For this review, take the finished solid that the model builds, in its own axes (mm). A direction names the side the tool comes from. Coordinates: 2 decimals unless noted, no trailing zeros. Loops run counter-clockwise (first coordinate to the right, second up) from the corner with the lowest first, then second, coordinate; pieces in that order, holes last. Notation, with made-up numbers: (-11, 2.25) -> (4, 2.25) arc R34 cw to (4, 41.25) -> close; hole circle Ø10 at (-21.75, 6). An arc over 180 degrees is marked (long way). Use a Markdown table: item, result.
from build123d import *

# Parameters (mm, degrees)
SKETCH1_R           = 4
BOSS_EXTRUDE1_DEPTH = 5
BOSS_EXTRUDE2_DEPTH = 35
SKETCH1_4_W         = 5
SKETCH1_4_H         = 35
BOSS_EXTRUDE3_DEPTH = 20
CHAMFER1_SIZE       = 8
CHAMFER1_SIZE2      = 21
FILLET1_R           = 25


with BuildPart() as part:
    # Sketch1 → Boss-Extrude1 (new body)
    with BuildSketch(Plane(origin=(0, 0, 0), x_dir=(1, 0, 0), z_dir=(0, 1, 0))):
        Polygon((5, -5), (5, -40), (60, -40), (75, -25), (75, -5), align=None)
        with Locations(Location((20, -25, 0), (0, 0, 270))):
            Circle(SKETCH1_R, mode=Mode.SUBTRACT)
        with Locations(Location((55, -25, 0), (0, 0, 270))):
            Circle(SKETCH1_R, mode=Mode.SUBTRACT)
    extrude(amount=BOSS_EXTRUDE1_DEPTH)

    # Sketch1_3 → Boss-Extrude2 (add)
    with BuildSketch(Plane(origin=(0, 0, 0), x_dir=(1, 0, 0), z_dir=(0, 1, 0))):
        Polygon((0, -5), (5, -5), (75, -5), (75, 0), (0, 0), align=None)
    extrude(amount=BOSS_EXTRUDE2_DEPTH)

    # Sketch1_4 → Boss-Extrude3 (add)
    with BuildSketch(Plane(origin=(0, 0, 0), x_dir=(1, 0, 0), z_dir=(0, 1, 0))):
        with Locations((2.5, -22.5)):
            Rectangle(SKETCH1_4_W, SKETCH1_4_H)
    extrude(amount=BOSS_EXTRUDE3_DEPTH)

    # Chamfer1
    chamfer1_edges = [part.edges().sort_by_distance(p)[0] for p in [
        (2.5, 20, 40),
    ]]
    chamfer1_side = [part.faces().sort_by_distance(p)[0] for p in [
        (24.5, 4.5, 40),
    ]]
    chamfer(chamfer1_edges, length=CHAMFER1_SIZE, length2=CHAMFER1_SIZE2, reference=chamfer1_side[0])

    # Fillet1
    fillet1_edges = [part.edges().sort_by_distance(p)[0] for p in [
        (75, 35, 2.5),
    ]]
    fillet(fillet1_edges, radius=FILLET1_R)


solid = part.part
(1) Mouldability with a two-part tool opening along X and no side actions: class faces 4 (the face through (40, 5, 22)), 5 (the face through (51.095, 2.465, 24.133)), 6 (the face through (0, 9, 16)) as pulls with the +X half, pulls with the -X half, needs draft (parallel to the pull), parting line crosses it, or undercut.
Found:
| item | result |
|---|---|
| face 4 | needs draft |
| face 5 | undercut |
| face 6 | pulls with the -X half |
(2) Take a section at A-A on x = 20. Write out the cut boundary in (y, z).
Found:
| item | result |
|---|---|
| outline | (0, 0) -> (35, 0) -> (35, 5) -> (5, 5) -> (5, 21) -> (0, 21) -> close; (0, 29) -> (5, 29) -> (5, 40) -> (0, 40) -> close |
(3) For line 1 along X through (y, z) = (2.35, 25); line 2 along Y through (x, z) = (50, 34.5), list the stretches that pass through material, from the lowest coordinate up.
Found:
| item | result |
|---|---|
| line 1 | x = 0 to 16, 24 to 51, 59 to 75 |
| line 2 | y = 0 to 5 |
(4) For faces 1 (the face through (25, 35, 2)), 2 (the face through (2, 20, 12)), 3 (the face through (5, 11, 23)), list the 3-axis set-ups (+Z, -Z, +X, -X, +Y, -Y) from which the entire face can be reached by the end or side of a thin tool; tool diameter is ignored.
Found:
| item | result |
|---|---|
| face 1 | +Z, -Z, +X, -X, +Y |
| face 2 | +Z, +X, -X, +Y |
| face 3 | +Z, +X, +Y |
(5) Take a section at B-B on z = 17. Write out the cut boundary in (x, y), plus the area to 3 significant figures.
Found:
| item | result |
|---|---|
| outline | (0, 0) -> (75, 0) -> (75, 5) -> (5, 5) -> (5, 20) -> (0, 20) -> close |
| area | 450 mm^2 |
(6) Take a section at C-C on x = 49. Write out the cut boundary in (y, z), plus the area to 3 significant figures.
Found:
| item | result |
|---|---|
| outline | (0, 0) -> (35, 0) -> (35, 5) -> (5, 5) -> (5, 40) -> (0, 40) -> close |
| area | 350 mm^2 |
(7) For pin 1 Ø4 at (x, z) = (3.5, 13) entering from +Y; pin 2 Ø3 at (x, z) = (15.5, 31.5) entering from +Y; pin 3 Ø10 at (x, y) = (53, 10.5) entering from +Z; pin 4 Ø5 at (x, y) = (51.5, 6) entering from -Z, all flat-tipped, find the tip position at first contact; note any pin that passes through.
Found:
| item | result |
|---|---|
| pin 1 | stops at y = 20 |
| pin 2 | stops at y = 5 |
| pin 3 | stops at z = 5 |
| pin 4 | stops at z = 0 |
(8) Take a section at D-D on z = 4. Write out the cut boundary in (x, y).
Found:
| item | result |
|---|---|
| outline | (0, 0) -> (75, 0) -> (75, 10) arc R25 ccw to (50, 35) -> (0, 35) -> close |
